The model under review builds one solid part; all positions refer to its coordinate system, in mm. A direction names the side the tool comes from. Coordinates: 2 decimals unless noted, no trailing zeros. Order: outer loops, then holes, each group sorted by start corner. A loop starts at its lowest first (then second) coordinate and runs counter-clockwise, first axis right, second up.
```python
from build123d import *

# Parameters (mm, degrees)
SKETCH2_R          = 3.9497
CUT_EXTRUDE1_DEPTH = 3.571875
SKETCH3_R          = 3.7703125
CUT_EXTRUDE2_DEPTH = 18.123368131
CUT_EXTRUDE3_START = -3.571875
SKETCH4_R          = 3.9497
CUT_EXTRUDE3_DEPTH = 3.571875


with BuildPart() as part:
    # Sketch1 → Revolve1 (revolve)
    with BuildSketch(Plane.XY, mode=Mode.PRIVATE) as revolve1_sk:
        Polygon((0, 0), (0, 4.7625), (-3.96875, 4.7625), (-3.96875, 4.76885), (-10.9982, 4.76885), (-10.9982, 6.35), (-14.5796, 6.35), (-14.5796, 0), align=None)
    revolve(revolve1_sk.sketch.rotate(Axis((-14.5796, 0, 0), (1, 0, 0)), 90), axis=Axis((-14.5796, 0, 0), (1, 0, 0)))

    # Sketch2 → Cut-Extrude1 (cut)
    with BuildSketch(Plane(origin=(0, 0, 0), x_dir=(0, 0, -1), z_dir=(1, 0, 0))):
        Circle(SKETCH2_R)
    extrude(amount=-CUT_EXTRUDE1_DEPTH, mode=Mode.SUBTRACT)

    # Sketch3 → Cut-Extrude2 (cut, through all)
    with BuildSketch(Plane.ZY.offset(14.5796)):
        Circle(SKETCH3_R)
    extrude(amount=-CUT_EXTRUDE2_DEPTH, mode=Mode.SUBTRACT)

    # Sketch4 → Cut-Extrude3 (cut)
    with BuildSketch(Plane.ZY.offset(14.5796).offset(CUT_EXTRUDE3_START)):
        with Locations(Location((0, 0, 0), (0, 0, 180))):
            Circle(SKETCH4_R)
    extrude(amount=CUT_EXTRUDE3_DEPTH, mode=Mode.SUBTRACT)


solid = part.part
```
(1) We need section C-C, the plane x = -2. Write out the cut boundary in (y, z) (1 decimal), and give its area (3 significant figures).
A:
outline: circle Ø9.5 at (0, 0); hole circle Ø7.9 at (0, 0)
area: 22.2 mm2
(2) Draft analysis for pull direction Z (two halves, no side actions). For faces 1 (the face through (-12.769, 3.856, 0.856)), 2 (the face through (-12.81, 3.86, -5.04)), 3 (the face through (-7.342, 0.166, -3.767)), 4 (the face through (-10.998, -5, -1)), state which applies: released by +Z, released by -Z, zero draft, split by the parting line, or undercut.
A:
face 1: undercut
face 2: split by the parting line
face 3: undercut
face 4: zero draft
(3) We need section D-D, the plane x = -11.5. Write out the cut boundary in (y, z), and give its area (3 significant figures).
A:
outline: circle Ø12.7 at (0, 0); hole circle Ø7.9 at (0, 0)
area: 77.7 mm2
(4) Machinability: for faces 5 (the face through (-14.58, -3, 3)), 6 (the face through (-1.761, 0.174, 3.946)), which of the approach directions +Z, -Z, +X, -X, +Y, -Y give a long, thin tool a straight path to every point of the face, cutting with its end or side? Answer none if there is none.
A:
face 5: +Z, -Z, -X, +Y, -Y
face 6: +X
(5) Wall thickness on probe 1 along Y at (x, z) = (-12.75, 0); probe 2 along Y at (x, z) = (-0.8, 0); probe 3 along X at (y, z) = (-1.5, 5.25): over which ranges is each line inside the solid? List them lowest first.
A:
probe 1: y = -6.35 to -3.95, 3.95 to 6.35
probe 2: y = -4.76 to -3.95, 3.95 to 4.76
probe 3: x = -14.58 to -11
(6) For pin 1 Ø6 at (x, y) = (-2, 3) entering from +Z; pin 2 Ø1.5 at (x, y) = (-4, -4) entering from -Z, all flat-tipped, find the tip position at first contact; note any pin that passes through.
A:
pin 1: stops at z = 4.76
pin 2: stops at z = -3.49
